from build123d import *

# Parameters (mm, degrees)
F2_W          = 94
F2_H          = 44
F3_DEPTH      = 203.2
F3_DEPTH_BACK = 205.74
F4_W          = 269.302904
F4_H          = 78
F5_DEPTH      = 10


with BuildPart() as f3:
    # F2 (on face) → F3 (new body, two sides)
    with BuildSketch(Plane(origin=(0, 0, 0), x_dir=(0.956305, 0, 0.292372), z_dir=(0.292372, 0, -0.956305))) as f3_sk:
        with BuildLine():
            ThreePointArc((-50, -22), (-49.12132, -24.12132), (-47, -25))
            Line((-47, -25), (47, -25))
            ThreePointArc((47, -25), (49.12132, -24.12132), (50, -22))
            Line((50, -22), (50, 22))
            ThreePointArc((50, 22), (49.12132, 24.12132), (47, 25))
            Line((47, 25), (-47, 25))
            ThreePointArc((-47, 25), (-49.12132, 24.12132), (-50, 22))
            Line((-50, 22), (-50, -22))
        make_face()
        Rectangle(F2_W, F2_H, mode=Mode.SUBTRACT)
    extrude(amount=F3_DEPTH)
    extrude(f3_sk.sketch, amount=-F3_DEPTH_BACK)

    # F4 (on face) → F5 (join)
    with BuildSketch(Plane(origin=(0, 25, 0), x_dir=(-1, 0, 0), z_dir=(0, 1, 0))):
        with Locations((-94.290361, 0)):
            Rectangle(F4_W, F4_H)
    extrude(amount=F5_DEPTH)


solid = f3.part
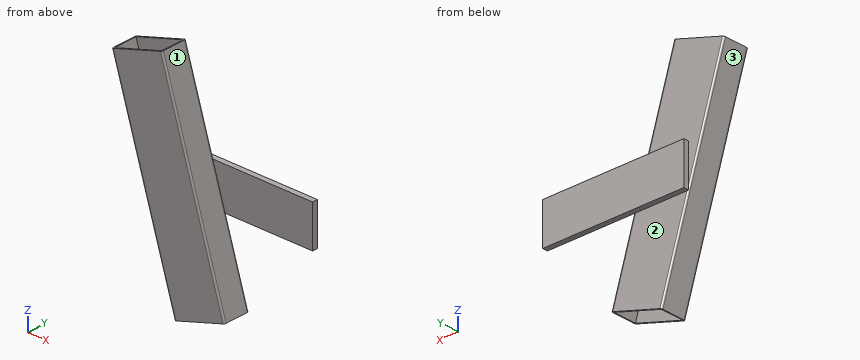
Source: CAD feature listing. Evaluate the final solid. Frame: model axes, mm. Face numbers are marked on the shaded views. A direction names the side the tool comes from. Give positions to 0.01 mm unless a question says otherwise; leave off trailing zeros. Write each loop counter-clockwise with the first axis right and the second up, starting at its lowest first coordinate (ties: lowest second). Pieces come first, ordered by that corner, then holes. Notation, with made-up numbers: (79, 11.5) -> (125, 11.5) arc R5 cw to (125, 20.5) -> close; hole circle Ø2 at (80, 39). An arc over 180 degrees is marked (long way). Return JSON: item names as keys, results as strings. Group by question number.
1. Section A-A, the plane y = 14. Output: boundary loops of the cut face in (x, z).
2. Material intervals for line 1 (Y direction, x = 49.5, z = -111); line 2 (Y direction, x = 165, z = 8.5); line 3 (X direction, y = -13, z = 99.5), sorted ascending. Write a range as from..to.
3. Access query for the marked faces 1, 2 and 3. Directions: +Z, -Z, +X, -X, +Y, -Y. A direction counts if a zero-diameter tool reaches every point of the face in a straight line with its end or side. Return the directions, or none.
4. Pin query (flat end, axial travel): pin 1 Ø3 at (x, y) = (129, 30.5) entering from -Z; pin 2 Ø8 at (y, z) = (30.5, 17) entering from -X; pin 3 Ø1 at (y, z) = (-9.5, 25.5) entering from +X; pin 4 Ø10 at (x, z) = (183.5, 45.5) entering from -Y. Return the tip coordinate at first contact, or that it passes through.
Determined:
{
 "1": {"outline": "(-107.97, 182.13) -> (11.59, -208.94) -> (14.46, -208.06) -> (-105.1, 183.01) -> close; (-15.21, 210.49) -> (104.36, -180.58) -> (107.23, -179.7) -> (-12.34, 211.37) -> close"},
 "2": {"line 1": "y = -25..-22, 22..25", "line 2": "y = 25..35", "line 3": "x = -82.7..-79.57, 18.73..21.86"},
 "3": {"face 1": "+Z, +X, -Y", "face 2": "-Z, +X, -X, +Y", "face 3": "-Z, -X, +Y, -Y"},
 "4": {"pin 1": "stops at z = -39", "pin 2": "stops at x = -40.36", "pin 3": "stops at x = 44.64", "pin 4": "passes through"}
}
